Here's how the part is built. I have some questions about the finished solid (model axes, mm). A direction names the side the tool comes from. Coordinates: 2 decimals unless noted, no trailing zeros. Loops run counter-clockwise (first coordinate to the right, second up) from the corner with the lowest first, then second, coordinate; pieces in that order, holes last. Notation, with made-up numbers: (82.5, 6.5) -> (105.5, 6.5) arc R32 ccw to (105.5, 41.5) -> close; hole circle Ø7 at (-32.75, -5.75). An arc over 180 degrees is marked (long way). Answer as a JSON object with one key per item and string values. Group by question number.
1) I need wall thicknesses on probe 1 along Z at (x, y) = (-19.25, 2.25); probe 2 along X at (y, z) = (6.5, 56.5); probe 3 along X at (y, z) = (2, 24.5). Which ranges of each line are inside material? Lowest first, please. Write a range as [from, to].
2) I want a section at B-B (y = 7). Count the separate pieces of the cut face and the enclosed holes in it, then the cut area to 3 significant figures.
3) Which directions (+Z, -Z, +X, -X, +Y, -Y) give clear straight access to the entire face, cutting with the end or side of a thin tool? Please do faces 3 (the flat face through (17, 5, 50)), 4 (the flat face through (-21, 0, 35)).
4) I want a section at C-C (x = 0). Write out the boundary of the cut face in (y, z), then the cut area to 3 significant figures.
5) I want a section at D-D (z = 30.5). Write out the boundary of the cut face in (x, y), then the cut area to 3 significant figures.
6) If we mould it in two halves opening along X, with no side actions, what happens to faces 1 (the flat face through (23.5, 8, 17)), 2 (the flat face through (0, 14, 70))? For each: +X half, -X half, draft (parallel to the pull), parting line (faces both ways), or undercut.
7) I want a section at A-A (z = 52.5). Write out the boundary of the cut face in (x, y), then the cut area to 3 significant figures.
8) I'm going to push flat-ended pins straight in: pin 1 (1 mm diameter, centred on y = 17.5, z = 47.5, fed in from +X); pin 2 (7.5 mm diameter, centred on x = -19.25, z = 17.5, fed in from +Y); pin 3 (5.5 mm diameter, centred on y = 12, z = 53.5, fed in from +X). Where does each tip first touch, or does it pass through?
```python
from build123d import *

# Parameters (mm, degrees)
PAD_DEPTH       = 70
SKETCH001_R     = 2.75
POCKET_DEPTH    = 25.251
SKETCH002_R     = 4.75
POCKET001_DEPTH = 20.251
FILLET_R        = 3


with BuildPart() as part:
    # Sketch → Pad (new body)
    with BuildSketch(Plane.XY):
        with BuildLine():
            ThreePointArc((14.716063, 0), (0, 13.75), (-14.716063, 0))
            Line((-26.230945, 0), (-14.716063, 0))
            ThreePointArc((26.230945, 0), (0, 25.25), (-26.230945, 0))
            Line((14.716063, 0), (26.230945, 0))
        make_face()
    extrude(amount=PAD_DEPTH)

    # Sketch001 (on Face2 of Pad) → Pocket (cut, through all)
    with BuildSketch(Plane.XZ):
        with Locations((-19.25, 17.5)):
            Circle(SKETCH001_R)
        with Locations((19.25, 17.5)):
            Circle(SKETCH001_R)
        with Locations((19.25, 52.5)):
            Circle(SKETCH001_R)
        with Locations((-19.25, 52.5)):
            Circle(SKETCH001_R)
    extrude(amount=-POCKET_DEPTH, mode=Mode.SUBTRACT)

    # Sketch002 (on DatumPlane) → Pocket001 (cut, through all)
    with BuildSketch(Plane.XZ.offset(-5)):
        with Locations((-19.25, 17.5)):
            Circle(SKETCH002_R)
        with Locations((-19.25, 52.5)):
            Circle(SKETCH002_R)
        Polygon((19.25, 12.592523), (23.5, 15.046261), (23.5, 19.953739), (19.25, 22.407477), (15, 19.953739), (15, 15.046261), align=None)
        Polygon((19.25, 47.592523), (23.5, 50.046261), (23.5, 54.953739), (19.25, 57.407477), (15, 54.953739), (15, 50.046261), align=None)
    extrude(amount=-POCKET001_DEPTH, mode=Mode.SUBTRACT)

    # Fillet
    fillet_edges = [part.edges().sort_by_distance(p)[0] for p in [
        (0, 25.25, 70),
    ]]
    fillet(fillet_edges, radius=FILLET_R)


solid = part.part
```
Determined:
{
 "1": {"probe 1": "[0, 14.75], [20.25, 49.75], [55.25, 70]", "probe 2": "[-25.16, -21.81], [-16.69, -12.7], [12.7, 17.68], [20.82, 25.16]", "probe 3": "[-26.08, -14.44], [14.44, 26.08]"},
 "2": {"separate pieces": "2", "enclosed holes": "4", "area": "1,490 mm^2"},
 "3": {"face 3": "+Y", "face 4": "+Z, -Z, +X, -X, -Y"},
 "4": {"outline": "(13.75, 0) -> (25.25, 0) -> (25.25, 67) arc R3 ccw to (22.25, 70) -> (13.75, 70) -> close", "area": "803 mm^2"},
 "5": {"outline": "(-26.23, 0) -> (-14.72, 0) arc R14.75 cw to (14.72, 0) -> (26.23, 0) arc R26.25 ccw to start", "area": "718 mm^2"},
 "6": {"face 1": "undercut", "face 2": "draft"},
 "7": {"outline": "(-26.23, 0) -> (-22, 0) -> (-22, 5) -> (-24, 5) -> (-24, 9.63) arc R26.25 ccw to start; (-16.5, 0) -> (-14.72, 0) arc R14.75 cw to (14.72, 0) -> (16.5, 0) -> (16.5, 5) -> (15, 5) -> (15, 20.54) arc R26.25 ccw to (-14.5, 20.88) -> (-14.5, 5) -> (-16.5, 5) -> close; (22, 0) -> (26.23, 0) arc R26.25 ccw to (23.5, 10.7) -> (23.5, 5) -> (22, 5) -> close", "area": "457 mm^2"},
 "8": {"pin 1": "x = 19.11", "pin 2": "y = 5", "pin 3": "x = 24.17"}
}
